from build123d import *

# Parameters (mm, degrees)
SKETCH1_R           = 2.5
BOSS_EXTRUDE1_DEPTH = 16
SKETCH2_R           = 1.25
BOSS_EXTRUDE2_DEPTH = 4.5
BOSS_EXTRUDE3_START = 1.5
SKETCH3_R           = 1.25
BOSS_EXTRUDE3_DEPTH = 1.5
SKETCH4_R           = 1.375
BOSS_EXTRUDE4_DEPTH = 1
FILLET1_R           = 0.75


with BuildPart() as part:
    # Sketch1 → Boss-Extrude1 (new body)
    with BuildSketch(Plane(origin=(0, 0, 0), x_dir=(1, 0, 0), z_dir=(0, 1, 0))):
        with Locations(Location((0, 0, 0), (0, 0, 270))):
            Circle(SKETCH1_R)
    extrude(amount=BOSS_EXTRUDE1_DEPTH)

    # Sketch2 → Boss-Extrude2 (add)
    with BuildSketch(Plane(origin=(0, 16, 0), x_dir=(1, 0, 0), z_dir=(0, 1, 0))):
        with Locations(Location((0, 0, 0), (0, 0, 270))):
            Circle(SKETCH2_R)
    extrude(amount=BOSS_EXTRUDE2_DEPTH)

    # Sketch3 → Boss-Extrude3 (add)
    with BuildSketch(Plane(origin=(0, 0, 0), x_dir=(-1, 0, 0), z_dir=(0, -1, 0)).offset(BOSS_EXTRUDE3_START)):
        with Locations(Location((0, 0, 0), (0, 0, 270))):
            Circle(SKETCH3_R)
    extrude(amount=-BOSS_EXTRUDE3_DEPTH)

    # Sketch4 → Boss-Extrude4 (add)
    with BuildSketch(Plane(origin=(0, -1.5, 0), x_dir=(-1, 0, 0), z_dir=(0, -1, 0))):
        with Locations(Location((0, 0, 0), (0, 0, 90))):
            Circle(SKETCH4_R)
    extrude(amount=BOSS_EXTRUDE4_DEPTH)

    # Fillet1
    fillet1_edges = [part.edges().sort_by_distance(p)[0] for p in [
        (0, -2.5, 1.375),
    ]]
    fillet(fillet1_edges, radius=FILLET1_R)


solid = part.part
Check sheet for the modelled part. Datum: model origin and axes. Units: mm. A direction names the side the tool comes from. Round coordinates to 2 decimals unless told otherwise and drop trailing zeros. Order: outer loops, then holes, each group sorted by start corner. A loop starts at its lowest first (then second) coordinate and runs counter-clockwise, first axis right, second up.
(1) Access from +Z, -Z, +X, -X, +Y, -Y to the whole of each face (thin tool, end or side, straight path). Record for faces 1 (the flat face through (0, -2.5, 0)), 2 (the flat face through (1, 16, 1)).
(2) Cross-section at C-C, the plane y = 9.5. Enter the section's corners in (x, z), and give its area (3 significant figures).
(3) Cross-section at B-B, the plane z = 2.05. Enter the section's corners in (x, y).
(4) Scan lines: probe 1 along Y at (x, z) = (-2.1, 0.3); probe 2 along Z at (x, y) = (-0.05, -0.25); probe 3 along X at (y, z) = (15.5, 0.1). Record each from-to range of solid material in increasing order.
(5) Draft check along Y on faces 3 (the flat face through (0, 20.5, 0)), 4 (the cylindrical face through (1.22, -0.76, -0.27)), 5 (the cylindrical face through (-1.22, 18.22, -0.27)). Enter one of: pulls with the +Y half, pulls with the -Y half, needs draft (parallel to the pull), parting line crosses it, or undercut.
(6) Cross-section at A-A, the plane y = 16.25. Enter the section's corners in (x, z), and give its area (3 significant figures).
(7) Go/stop test with flat-tipped pins: P1, Ø1, axis at x = 1, y = 3.5, coming from the +Z side; P2, Ø3, axis at x = -2, z = 2, coming from the +Y side. Record where each tip stops, or that it passes through.
Check sheet entries:
1. face 1: +Z, -Z, +X, -X, -Y
1. face 2: +Y
2. outline: circle Ø5 at (0, 0)
2. area: 19.6 mm2
3. outline: (-1.43, 0) - (1.43, 0) - (1.43, 16) - (-1.43, 16) - close
4. probe 1: y = 0 to 16
4. probe 2: z = -1.25 to 1.25
4. probe 3: x = -2.5 to 2.5
5. face 3: pulls with the +Y half
5. face 4: undercut
5. face 5: needs draft
6. outline: circle Ø2.5 at (0, 0)
6. area: 4.91 mm2
7. P1: stops at z = 2.45
7. P2: stops at y = 16
